Read the model definition and answer for the solid it produces. Units are mm, in the model's axes. A direction names the side the tool comes from. Give positions to 0.01 mm unless a question says otherwise; leave off trailing zeros. Order: outer loops, then holes, each group sorted by start corner. A loop starts at its lowest first (then second) coordinate and runs counter-clockwise, first axis right, second up.
```python
from build123d import *

# Parameters (mm, degrees)
F0_W     = 130
F0_H     = 60
F0_W_2   = 124
F0_H_2   = 54
F1_DEPTH = 44
F2_R     = 2
F2_R_2   = 1
F3_DEPTH = 60.001
F4_W     = 124
F4_H     = 54
F5_DEPTH = 3


with BuildPart() as f1:
    # F0 (on Top) → F1 (new body)
    with BuildSketch(Plane.XY):
        Rectangle(F0_W, F0_H)
        Rectangle(F0_W_2, F0_H_2, mode=Mode.SUBTRACT)
    extrude(amount=F1_DEPTH)

    # F2 (on face) → F3 (cut, through all)
    with BuildSketch(Plane.XZ.offset(30)):
        with Locations((55, 10)):
            Circle(F2_R)
        with Locations((-55, 10)):
            Circle(F2_R)
        with Locations((0, 24)):
            Circle(F2_R)
        with Locations((0, 34)):
            Circle(F2_R_2)
    extrude(amount=-F3_DEPTH, mode=Mode.SUBTRACT)

    # F4 (on Top) → F5 (join)
    with BuildSketch(Plane.XY):
        Rectangle(F4_W, F4_H)
    extrude(amount=F5_DEPTH)


solid = f1.part
```
1) The part is cut by section D-D on y = 23. Determine the outline of the cut face in (x, z), and give its area (3 significant figures).
Final values:
outline: (-65, 0) - (65, 0) - (65, 44) - (62, 44) - (62, 3) - (-62, 3) - (-62, 44) - (-65, 44) - close
area: 636 mm2
2) The part is cut by section A-A on z = 24. Determine the outline of the cut face in (x, y).
Final values:
outline: (-65, -30) - (-2, -30) - (-2, -27) - (-62, -27) - (-62, 27) - (-2, 27) - (-2, 30) - (-65, 30) - close; (2, -30) - (65, -30) - (65, 30) - (2, 30) - (2, 27) - (62, 27) - (62, -27) - (2, -27) - close
3) For a pull along X with two mould halves and no side action, classify faces 3 (the face through (65, 0, 22)), 4 (the face through (0.923, -28.521, 22.226)), 5 (the face through (-65, 0, 22)), 6 (the face through (-5, -29, 44)) as released by +X, released by -X, zero draft, split by the parting line, or undercut.
Final values:
face 3: released by +X
face 4: undercut
face 5: released by -X
face 6: zero draft
4) The part is cut by section C-C on z = 15. Determine the outline of the cut face in (x, y).
Final values:
outline: (-65, -30) - (65, -30) - (65, 30) - (-65, 30) - close; hole (-62, -27) - (62, -27) - (62, 27) - (-62, 27) - close
5) The part is cut by section B-B on x = 19.5. Determine the outline of the cut face in (y, z).
Final values:
outline: (-30, 0) - (30, 0) - (30, 44) - (27, 44) - (27, 3) - (-27, 3) - (-27, 44) - (-30, 44) - close
6) Given pin 1 (2.5 mm diameter, centred on x = -55, z = 10, fed in from +Y); pin 2 (10 mm diameter, centred on x = 19.5, y = -13, fed in from +Z), each flat-ended and moving along its own axis, determine where each tip first touches the part or whether it passes through.
Final values:
pin 1: passes through
pin 2: stops at z = 3
7) A tool of negligible diameter and unlimited length cuts with its end or side. For faces 1 (the face through (-62, 0, 23)), 2 (the face through (0.923, 28.479, 22.226)), from which of +Z, -Z, +X, -X, +Y, -Y can it reach the whole face along a straight path? Write none if from no direction.
Final values:
face 1: +Z
face 2: +Y, -Y
8) Consider L1, parallel to Z at x = 0, y = 29.1; L2, parallel to Y at x = -11, z = 13; L3, parallel to X at y = 26, z = 23. Determine where each line is inside the solid, lowest interval first.
Final values:
L1: z = 0 to 22, 26 to 33, 35 to 44
L2: y = -30 to -27, 27 to 30
L3: x = -65 to -62, 62 to 65
